Geometry check sheet. Reference: the model listing, model coordinates, mm. A direction names the side the tool comes from. Coordinates: 2 decimals unless noted, no trailing zeros. Loops run counter-clockwise (first coordinate to the right, second up) from the corner with the lowest first, then second, coordinate; pieces in that order, holes last. Notation, with made-up numbers: (40.25, -20.75) - (98.25, -20.75) arc R27 ccw to (98.25, 2.25) - close; hole circle Ø9 at (7.25, 28.25). An arc over 180 degrees is marked (long way). One line per item, written item: value.
from build123d import *

# Parameters (mm, degrees)
SALIENTE_EXTRUIR1_DEPTH    = 190
CROQUIS3_W                 = 56.281965067
CROQUIS3_H                 = 32
CORTAR_EXTRUIR1_DEPTH      = 25.039324
CORTAR_EXTRUIR3_DEPTH      = 25.039324
SALIENTE_EXTRUIR2_REACH    = 62
SALIENTE_EXTRUIR3_REACH    = 132
CROQUIS7_W                 = 4
CROQUIS7_H                 = 12
CORTAR_EXTRUIR6_DEPTH      = 30
CROQUIS8_R                 = 1.25
CORTAR_EXTRUIR7_DEPTH      = 18
CORTAR_EXTRUIR7_DEPTH_BACK = 14.03932438
CROQUIS9_R                 = 3.5
CORTAR_EXTRUIR8_DEPTH      = 8


with BuildPart() as part:
    # Croquis1 → Saliente-Extruir1 (new body)
    with BuildSketch(Plane.XY):
        with BuildLine():
            Line((56.281965067, 0), (27.121320344, 29.160644724))
            ThreePointArc((27.121320344, 29.160644724), (26.148050297, 29.810962978), (25, 30.03932438))
            Line((25, 30.03932438), (0, 30.03932438))
            Line((0, 30.03932438), (0, 0))
            Line((0, 0), (56.281965067, 0))
        make_face()
    extrude(amount=SALIENTE_EXTRUIR1_DEPTH)

    # Croquis3 → Cortar-Extruir1 (cut)
    with BuildSketch(Plane.XZ):
        with Locations((28.140982534, 146)):
            Rectangle(CROQUIS3_W, CROQUIS3_H)
        with Locations((28.140982534, 44)):
            Rectangle(CROQUIS3_W, CROQUIS3_H)
    extrude(amount=-CORTAR_EXTRUIR1_DEPTH, mode=Mode.SUBTRACT)

    # Croquis4 → Cortar-Extruir3 (cut)
    with BuildSketch(Plane.XZ):
        Polygon((0, 130), (15, 130), (7.928932188, 122.928932188), (7.928932188, 67.071067812), (15, 60), (0, 60), align=None)
    extrude(amount=-CORTAR_EXTRUIR3_DEPTH, mode=Mode.SUBTRACT)

    # Croquis5 → Saliente-Extruir2 (add, up to next)
    with BuildSketch(Plane.XY.offset(130), mode=Mode.PRIVATE) as saliente_extruir2_sk1:
        Polygon((56.281965067, 0), (0, 0), (0, 13.03932438), (43.242640687, 13.03932438), align=None)
    saliente_extruir2_tool1 = extrude(saliente_extruir2_sk1.sketch, amount=SALIENTE_EXTRUIR2_REACH, mode=Mode.PRIVATE) - part.part
    add(saliente_extruir2_tool1.solids().sort_by_distance((25.023515, 6.234935, 130))[0])

    # Croquis6 → Saliente-Extruir3 (add, up to next)
    with BuildSketch(Plane(origin=(0, 0, 130), x_dir=(-1, 0, 0), z_dir=(0, 0, -1)), mode=Mode.PRIVATE) as saliente_extruir3_sk1:
        Polygon((0, 0), (0, 13.03932438), (-43.242640687, 13.03932438), (-56.281965067, 0), align=None)
    saliente_extruir3_tool1 = extrude(saliente_extruir3_sk1.sketch, amount=SALIENTE_EXTRUIR3_REACH, mode=Mode.PRIVATE) - part.part
    add(saliente_extruir3_tool1.solids().sort_by_distance((25.023515, 6.234935, 130))[0])

    # Croquis7 → Cortar-Extruir6 (cut)
    with BuildSketch(Plane.ZY):
        with Locations((26, 19.03932438)):
            Rectangle(CROQUIS7_W, CROQUIS7_H)
        with Locations((164, 19.03932438)):
            Rectangle(CROQUIS7_W, CROQUIS7_H)
    extrude(amount=-CORTAR_EXTRUIR6_DEPTH, mode=Mode.SUBTRACT)

    # Croquis8 → Cortar-Extruir7 (cut, two sides)
    with BuildSketch(Plane(origin=(0, 13.03932438, 0), x_dir=(1, 0, 0), z_dir=(0, 1, 0))) as cortar_extruir7_sk:
        with Locations((20.242640687, -158.7)):
            Circle(CROQUIS8_R)
        with Locations((20.242640687, -133.3)):
            Circle(CROQUIS8_R)
        with Locations((20.242640687, -31.3)):
            Circle(CROQUIS8_R)
        with Locations((20.242640687, -56.7)):
            Circle(CROQUIS8_R)
    extrude(amount=CORTAR_EXTRUIR7_DEPTH, mode=Mode.SUBTRACT)
    extrude(cortar_extruir7_sk.sketch, amount=-CORTAR_EXTRUIR7_DEPTH_BACK, mode=Mode.SUBTRACT)

    # Croquis9 → Cortar-Extruir8 (cut)
    with BuildSketch(Plane.XZ):
        with Locations((20.242640687, 158.7)):
            Circle(CROQUIS9_R)
        with Locations((20.242640687, 133.3)):
            Circle(CROQUIS9_R)
        with Locations((20.242640687, 56.7)):
            Circle(CROQUIS9_R)
        with Locations((20.242640687, 31.3)):
            Circle(CROQUIS9_R)
    extrude(amount=-CORTAR_EXTRUIR8_DEPTH, mode=Mode.SUBTRACT)


solid = part.part
(1) Cross-section at C-C on y = 16. Record the cut outline in (x, z).
Reply:
outline: (0, 0) - (40.28, 0) - (40.28, 28) - (30, 28) - (30, 24) - (0, 24) - close; (0, 166) - (30, 166) - (30, 162) - (40.28, 162) - (40.28, 190) - (0, 190) - close; (7.93, 67.07) - (15, 60) - (40.28, 60) - (40.28, 130) - (15, 130) - (7.93, 122.93) - close
(2) Go/stop test with flat-tipped pins: pin 1 Ø5 at (x, z) = (27.5, 107.5) entering from +Y; pin 2 Ø8 at (y, z) = (20.5, 55.5) entering from +X; pin 3 Ø3 at (x, z) = (30.5, 33) entering from +Y; pin 4 Ø10 at (x, z) = (50, 152) entering from +Y. Record where each tip stops, or that it passes through.
Reply:
pin 1: y = 30.04
pin 2: through
pin 3: y = 27.28
pin 4: y = 11.28
(3) Access from +Z, -Z, +X, -X, +Y, -Y to the whole of each face (thin tool, end or side, straight path). Record for faces 4 (the face through (11, 19, 64)), 5 (the face through (0, 11, 96)), 6 (the face through (19.484, 3.944, 27.883)), 7 (the face through (26, 19, 130)).
Reply:
face 4: -X
face 5: +Z, -Z, -X, +Y, -Y
face 6: -Y
face 7: +X, -X
(4) Release check for a two-part mould opening along Y. For faces 1 (the face through (30, 19, 164)), 2 (the face through (13, 30.039, 94)), 3 (the face through (21, 12, 190)) record: pulls with the +Y half, pulls with the -Y half, needs draft (parallel to the pull), parting line crosses it, or undercut.
Reply:
face 1: undercut
face 2: pulls with the +Y half
face 3: needs draft
(5) Cross-section at D-D on x = 50. Record the cut outline in (y, z).
Reply:
outline: (0, 0) - (6.28, 0) - (6.28, 190) - (0, 190) - close
(6) Cross-section at A-A on z = 51.5. Record the cut outline in (x, y), and give its area (3 significant figures).
Reply:
outline: (0, 0) - (56.28, 0) - (43.24, 13.04) - (0, 13.04) - close; (0, 25.04) - (31.24, 25.04) - (27.12, 29.16) arc R3 ccw to (25, 30.04) - (0, 30.04) - close
area: 792 mm2
(7) Cross-section at B-B on y = 6. Record the cut outline in (x, z), and give its area (3 significant figures).
Reply:
outline: (0, 0) - (50.28, 0) - (50.28, 190) - (0, 190) - close; hole circle Ø7 at (20.24, 31.3); hole circle Ø7 at (20.24, 56.7); hole circle Ø7 at (20.24, 133.3); hole circle Ø7 at (20.24, 158.7)
area: 9,400 mm2
(8) Material ranges on probe 1 along Z at (x, y) = (24, 18); probe 2 along Z at (x, y) = (35, 14.5); probe 3 along Y at (x, z) = (7.5, 146.5), recorded low to high. Write a range as from..to.
Reply:
probe 1: 0..24, 60..130, 166..190
probe 2: 0..28, 60..130, 162..190
probe 3: 0..13.04, 25.04..30.04
